Build history of the part. All positions in model axes, mm. Face numbers are marked on the shaded views. A direction names the side the tool comes from. Give positions to 0.01 mm unless a question says otherwise; leave off trailing zeros. Order: outer loops, then holes, each group sorted by start corner. A loop starts at its lowest first (then second) coordinate and runs counter-clockwise, first axis right, second up. Notation, with made-up numbers: (46.25, 81.25) - (66.25, 81.25) arc R29 cw to (66.25, 114.25) - close; hole circle Ø4 at (5, 10). An arc over 180 degrees is marked (long way). Write each question's results on one line, items separated by ' | '. Start each with the question number.
from build123d import *
from build123d.topology import SkipClean

# Parameters (mm, degrees)
BOSS_EXTRUDE1_START           = 5
BOSS_EXTRUDE1_DEPTH           = 6
CHAMFER1_SIZE                 = 4.5
SKETCH2_W                     = 6
SKETCH2_H                     = 6.3
BOSS_EXTRUDE2_DEPTH           = 6.3
BOSS_EXTRUDE3_DEPTH           = 7.3
BOSS_EXTRUDE4_DEPTH           = 14.405295
CSK_FOR_M3_SFHCS1_D           = 3
CSK_FOR_M3_SFHCS1_CSINK_D     = 6.3
CSK_FOR_M3_SFHCS1_CSINK_ANGLE = 90
CSK_FOR_M3_SFHCS2_D           = 3
CSK_FOR_M3_SFHCS2_CSINK_D     = 6.3
CSK_FOR_M3_SFHCS2_CSINK_ANGLE = 90


with BuildPart() as part:
    # Sketch1 → Boss-Extrude1 (new body)
    with BuildSketch(Plane.XY.offset(BOSS_EXTRUDE1_START)):
        with BuildLine():
            Line((-23.5, -12), (-7, -12))
            Line((-7, -12), (-7, -8.5))
            ThreePointArc((-7, -8.5), (-6.853553391, -8.146446609), (-6.5, -8))
            Line((-6.5, -8), (6.5, -8))
            ThreePointArc((6.5, -8), (6.853553391, -8.146446609), (7, -8.5))
            Line((7, -8.5), (7, -12))
            Line((7, -12), (23.5, -12))
            Line((23.5, -12), (26, -9.5))
            Line((26, -9.5), (26, -3.15))
            Line((26, -3.15), (32.3, -3.15))
            Line((32.3, -3.15), (32.3, 3.15))
            Line((32.3, 3.15), (26, 3.15))
            Line((26, 3.15), (26, 9.5))
            Line((26, 9.5), (23.5, 12))
            Line((23.5, 12), (6, 12))
            Line((6, 12), (6, 5.5))
            ThreePointArc((6, 5.5), (5.853553391, 5.146446609), (5.5, 5))
            Line((5.5, 5), (-5.5, 5))
            ThreePointArc((-5.5, 5), (-5.853553391, 5.146446609), (-6, 5.5))
            Line((-6, 5.5), (-6, 12))
            Line((-6, 12), (-23.5, 12))
            Line((-23.5, 12), (-26, 9.5))
            Line((-26, 9.5), (-26, 3.15))
            Line((-26, 3.15), (-32.3, 3.15))
            Line((-32.3, 3.15), (-32.3, -3.15))
            Line((-32.3, -3.15), (-26, -3.15))
            Line((-26, -3.15), (-26, -9.5))
            Line((-26, -9.5), (-23.5, -12))
        make_face()
    extrude(amount=BOSS_EXTRUDE1_DEPTH)

    # Chamfer1
    chamfer1_edges = [part.edges().sort_by_distance(p)[0] for p in [
        (7, -10.25, 5),
        (6.853553391, -8.146446609, 5),
        (0, -8, 5),
        (-6.853553391, -8.146446609, 5),
        (-7, -10.25, 5),
    ]]
    chamfer(chamfer1_edges, length=CHAMFER1_SIZE)

    # Sketch2 → Boss-Extrude2 (add)
    with BuildSketch(Plane(origin=(26, 0, 0), x_dir=(0, 0, -1), z_dir=(1, 0, 0))):
        with Locations((-8, 0)):
            Rectangle(SKETCH2_W, SKETCH2_H)
    boss_extrude2 = extrude(amount=BOSS_EXTRUDE2_DEPTH)

    # Mirror1: Boss-Extrude2 across plane
    add(boss_extrude2.mirror(Plane(origin=(0, 0, 0), x_dir=(0, 0, 1), z_dir=(1, 0, 0))))

    # Sketch3 → Boss-Extrude3 (add)
    with BuildSketch(Plane.XY.offset(11)):
        Polygon((11.551404138, 1.816830905), (2.291859281, -9.218264944), (8.439052056, -14.376372134), (17.698596913, -3.341276285), align=None)
    extrude(amount=BOSS_EXTRUDE3_DEPTH)

    # Sketch4 → Boss-Extrude4 (add)
    with SkipClean():  # the faces are left unmerged after this step: merging them gives an invalid solid
        with BuildSketch(Plane(origin=(5.667376511, 6.754116317, 0), x_dir=(0.7660444431189792, -0.6427876096865379, 0), z_dir=(0.6427876096865379, 0.7660444431189792, 0))):
            with BuildLine():
                Line((15.705642813, -18.3), (7.681052555, -18.3))
                ThreePointArc((7.681052555, -18.3), (11.693347684, -22.312295129), (15.705642813, -18.3))
            make_face()
        extrude(amount=-BOSS_EXTRUDE4_DEPTH)

    # CSK for M3 SFHCS1 (through all)
    with Locations(Plane(origin=(5.667376511, 6.754116317, 0), x_dir=(0.7660444431189792, -0.6427876096865379, 0), z_dir=(0.6427876096865379, 0.7660444431189792, 0))):
        with Locations((11.693347684, -18.3)):
            CounterSinkHole(CSK_FOR_M3_SFHCS1_D / 2, CSK_FOR_M3_SFHCS1_CSINK_D / 2, counter_sink_angle=CSK_FOR_M3_SFHCS1_CSINK_ANGLE)

    # CSK for M3 SFHCS2 (through all)
    with Locations(Plane(origin=(-1490.377712475, -7.825775805, -12), x_dir=(-0.766044443118981, 0.6427876096865359, 0), z_dir=(0, 0, -1))):
        with Locations((-1114.335057549, 945.253960578), (-1158.995448583, 982.728478223)):
            CounterSinkHole(CSK_FOR_M3_SFHCS2_D / 2, CSK_FOR_M3_SFHCS2_CSINK_D / 2, counter_sink_angle=CSK_FOR_M3_SFHCS2_CSINK_ANGLE)


solid = part.part
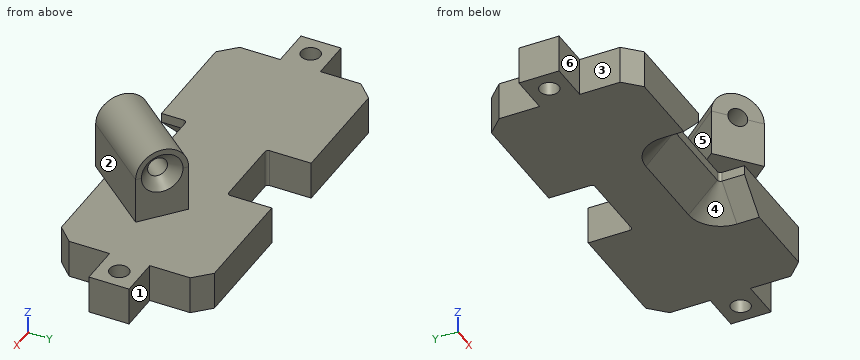
Item 1: Two-plate mould, pull along X, no slides. Class the marked faces 4, 5 and 6: +X half, -X half, draft (parallel to the pull), parting line (faces both ways), or undercut.
Item 2: Cut at D-D, the plane x = -20. List the corners of the cut face in (y, z), then the cut area to 3 significant figures.
Item 3: Cut at B-B, the plane y = 2.5. List the corners of the cut face in (x, z).
Item 4: Cut at A-A, the plane x = 29.15. List the corners of the cut face in (y, z).
Item 5: Flat gauge pins, fed straight in: pin 1 Ø2 at (x, y) = (-24.5, -7) entering from +Z; pin 2 Ø5 at (x, z) = (-11.5, 7.5) entering from -Y; pin 3 Ø1.5 at (y, z) = (-4.5, 14) entering from +X; pin 4 Ø5 at (y, z) = (5, 8.5) entering from +X. Where does each tip first touch, or does it go through?
Item 6: Probe line 1 along X through (y, z) = (0, 9.4); line 2 along Y through (x, z) = (-29.15, 9.5); line 3 along X through (y, z) = (7.5, 7). List the from-to ranges inside material, lowest first. Write a range as from..to.
Item 7: Which spindle directions (+Z, -Z, +X, -X, +Y, -Y) get a long thin tool onto all of the face, cutting with end or side? Do the marked faces 1, 2 and 3. Say none if no direction does.
Item 8: Cut at C-C, the plane x = -4. List the corners of the cut face in (y, z).
Values found:
1) face 4: undercut | face 5: -X half | face 6: draft
2) outline: (-12, 5) - (12, 5) - (12, 11) - (-12, 11) - close | area: 144 mm2
3) outline: (-32.3, 5) - (32.3, 5) - (32.3, 11) - (-32.3, 11) - close
4) outline: (-3.15, 5) - (-1.5, 5) - (-1.5, 11) - (-3.15, 11) - close; (1.5, 5) - (3.15, 5) - (3.15, 11) - (1.5, 11) - close
5) pin 1: stops at z = 11 | pin 2: stops at y = -12 | pin 3: stops at x = 17.36 | pin 4: stops at x = 32.3
6) line 1: x = -32.3..-30.65, -27.65..27.65, 30.65..32.3 | line 2: y = -3.15..-1.5, 1.5..3.15 | line 3: x = -26..-6, 6..26
7) face 1: +Z, -Z, +X, +Y | face 2: +Z, +X, -Y | face 3: +Z, -Z, -X, -Y
8) outline: (-8, 9.5) - (-3.5, 5) - (5, 5) - (5, 11) - (-8, 11) - close
